```python
from build123d import *

# Parameters (mm, degrees)
SKETCH1_W           = 45
SKETCH1_H           = 45
BOSS_EXTRUDE1_DEPTH = 40
SKETCH2_W           = 45
SKETCH2_H           = 70
BOSS_EXTRUDE2_DEPTH = 20
CHAMFER1_SIZE       = 15
CHAMFER2_SIZE       = 35
SKETCH3_R           = 20
CUT_EXTRUDE1_DEPTH  = 25
SKETCH4_W           = 40
SKETCH4_H           = 20
CUT_EXTRUDE2_DEPTH  = 49


with BuildPart() as part:
    # Sketch1 → Boss-Extrude1 (new body)
    with BuildSketch(Plane(origin=(0, 0, 0), x_dir=(1, 0, 0), z_dir=(0, 1, 0))):
        Rectangle(SKETCH1_W, SKETCH1_H)
    extrude(amount=BOSS_EXTRUDE1_DEPTH)

    # Sketch2 → Boss-Extrude2 (add)
    with BuildSketch(Plane(origin=(0, 40, 0), x_dir=(1, 0, 0), z_dir=(0, 1, 0))):
        with Locations((0, -12.5)):
            Rectangle(SKETCH2_W, SKETCH2_H)
    extrude(amount=BOSS_EXTRUDE2_DEPTH)

    # Chamfer1
    chamfer1_edges = [part.edges().sort_by_distance(p)[0] for p in [
        (0, 40, 22.5),
    ]]
    chamfer(chamfer1_edges, length=CHAMFER1_SIZE)

    # Chamfer2
    chamfer2_edges = [part.edges().sort_by_distance(p)[0] for p in [
        (0, 60, -22.5),
    ]]
    chamfer(chamfer2_edges, length=CHAMFER2_SIZE)

    # Sketch3 → Cut-Extrude1 (cut)
    with BuildSketch(Plane(origin=(0, 0, 0), x_dir=(1, 0, 0), z_dir=(0, 1, 0))):
        with Locations(Location((0, 0, 0), (0, 0, 270))):
            Circle(SKETCH3_R)
    extrude(amount=CUT_EXTRUDE1_DEPTH, mode=Mode.SUBTRACT)

    # Sketch4 → Cut-Extrude2 (cut)
    with BuildSketch(Plane(origin=(0, 1.414213562, 1.414213562), x_dir=(-1, 0, 0), z_dir=(0, 0.7071067811865476, 0.7071067811865476))):
        with Locations((0, -21.587572106)):
            Rectangle(SKETCH4_W, SKETCH4_H)
    extrude(amount=CUT_EXTRUDE2_DEPTH, mode=Mode.SUBTRACT)


solid = part.part
```
CAD build for the part. Positions are in the model's coordinates, mm. A direction names the side the tool comes from. Give positions to 0.01 mm unless a question says otherwise; leave off trailing zeros. Loops run counter-clockwise (first coordinate to the right, second up) from the corner with the lowest first, then second, coordinate; pieces in that order, holes last. Notation, with made-up numbers: (87, 15) - (122, 15) arc R31 cw to (122, 46) - close; hole circle Ø7 at (68, 3). An arc over 180 degrees is marked (long way). Put each result on its own line as item: value.
Q1. Tool access for faces 1 (the face through (-20, 34, 3)), 2 (the face through (0, 12, 22.5)), 3 (the face through (0, 25, 13)): list every direction of +Z, -Z, +X, -X, +Y, -Y with a clear straight run to the whole face (end or side of a thin tool).
Filled in:
face 1: none
face 2: +Z, +X, -X, -Y
face 3: -Y
Q2. Slice it at D-D (y = 6). Give the cut face in (x, z).
Filled in:
outline: (-22.5, -22.5) - (22.5, -22.5) - (22.5, 22.5) - (-22.5, 22.5) - close; hole circle Ø40 at (0, 0)
Q3. Flat gauge pins, fed straight in: pin 1 (3 mm diameter, centred on x = -11.5, y = 6.5, fed in from +Z); pin 2 (3 mm diameter, centred on x = -13, y = 48, fed in from -Z); pin 3 (10 mm diameter, centred on x = 6.5, y = 38.5, fed in from +Z); pin 4 (3.5 mm diameter, centred on x = 1.5, z = 15, fed in from -Y). Where does each tip first touch, or does it go through?
Filled in:
pin 1: stops at z = 22.5
pin 2: stops at z = -1
pin 3: stops at z = 47.5
pin 4: stops at y = 25
Q4. Slice it at A-A (y = 18.5). Give the cut face in (x, z).
Filled in:
outline: (-22.5, -22.5) - (22.5, -22.5) - (22.5, 22.5) - (-22.5, 22.5) - close; hole (-20, -15.67) - (-12.43, -15.67) arc R20 ccw to (12.43, -15.67) - (20, -15.67) - (20, 2.11) - (19.89, 2.11) arc R20 ccw to (-19.89, 2.11) - (-20, 2.11) - close
Q5. Slice it at C-C (z = -4). Give the cut face in (x, y), plus the area to 3 significant figures.
Filled in:
outline: (-22.5, 0) - (-19.6, 0) - (-19.6, 12.39) - (-20, 12.39) - (-20, 40.67) - (20, 40.67) - (20, 12.39) - (19.6, 12.39) - (19.6, 0) - (22.5, 0) - (22.5, 43.5) - (-22.5, 43.5) - close
area: 341 mm²
Q6. Slice it at B-B (x = 0). Give the cut face in (y, z), plus the area to 3 significant figures.
Filled in:
outline: (0, -22.5) - (25, -22.5) - (60, 12.5) - (60, 47.5) - (40, 47.5) - (40, 37.5) - (25, 22.5) - (0, 22.5) - (0, 20) - (25, 20) - (25, 8.61) - (44.26, 27.87) - (58.4, 13.73) - (25, -19.67) - (25, -20) - (24.67, -20) - (23.75, -20.92) - (22.83, -20) - (0, -20) - close
area: 955 mm²
Q7. Mould opens along Y. For faces 4 (the face through (0.28, 40.83, -3.84)), 5 (the face through (0, 60, 30)), 6 (the face through (0, 40, 42)) say: pulls with the +Y half, pulls with the -Y half, needs draft (parallel to the pull), parting line crosses it, or undercut.
Filled in:
face 4: undercut
face 5: pulls with the +Y half
face 6: pulls with the -Y half
Q8. Probe line 1 along X through (y, z) = (12, 0); line 2 along X through (y, z) = (12.5, 10). List the from-to ranges inside material, lowest first.
Filled in:
line 1: x = -22.5 to -20, 20 to 22.5
line 2: x = -22.5 to -17.32, 17.32 to 22.5
